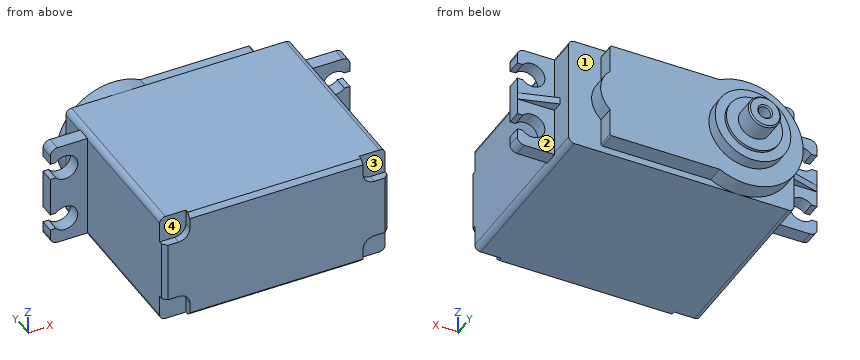
```python
from build123d import *

# Parameters (mm, degrees)
BOSS_EXTRUDE1_DEPTH = 33.6042
CUT_EXTRUDE1_DEPTH  = 1.397
CHAMFER1_SIZE       = 0.762
SKETCH3_W           = 18.6436
SKETCH3_H           = 2.4892
BOSS_EXTRUDE2_DEPTH = 6.604
SKETCH4_W           = 18.6436
SKETCH4_H           = 2.4892
BOSS_EXTRUDE3_DEPTH = 6.604
FILLET1_R           = 1.27
CUT_EXTRUDE2_DEPTH  = 3.048
SKETCH6_W           = 6.604
SKETCH6_H           = 1.2192
BOSS_EXTRUDE4_DEPTH = 1.905
CUT_EXTRUDE3_DEPTH  = 1.905
BOSS_EXTRUDE5_DEPTH = 3.0988
SKETCH9_R           = 6.731
BOSS_EXTRUDE6_DEPTH = 2.159
SKETCH10_R          = 4.9911
BOSS_EXTRUDE7_DEPTH = 0.508
SKETCH11_R          = 2.8702
BOSS_EXTRUDE8_DEPTH = 3.6576
SKETCH12_R          = 1.0668
CUT_EXTRUDE4_DEPTH  = 5.08
CHAMFER2_SIZE       = 0.254


with BuildPart() as part:
    # Sketch1 → Boss-Extrude1 (new body)
    with BuildSketch(Plane(origin=(0, 0, 0), x_dir=(1, 0, 0), z_dir=(0, 1, 0))):
        with BuildLine():
            Line((0, 9.0424), (0, -9.0424))
            ThreePointArc((0, -9.0424), (0.29757951, -9.76082049), (1.016, -10.0584))
            Line((1.016, -10.0584), (39.116, -10.0584))
            ThreePointArc((39.116, -10.0584), (39.83442049, -9.76082049), (40.132, -9.0424))
            Line((40.132, -9.0424), (40.132, 9.0424))
            ThreePointArc((40.132, 9.0424), (39.83442049, 9.76082049), (39.116, 10.0584))
            Line((39.116, 10.0584), (1.016, 10.0584))
            ThreePointArc((1.016, 10.0584), (0.29757951, 9.76082049), (0, 9.0424))
        make_face()
    extrude(amount=BOSS_EXTRUDE1_DEPTH)

    # Sketch2 → Cut-Extrude1 (cut)
    with BuildSketch(Plane.XZ):
        with BuildLine():
            Line((4.6482, 10.0584), (4.6482, 7.3533))
            ThreePointArc((4.6482, 7.3533), (4.067919955, 5.952380045), (2.667, 5.3721))
            Line((2.667, 5.3721), (0, 5.3721))
            Line((0, 5.3721), (0, 9.0424))
            ThreePointArc((0, 9.0424), (0.29757951, 9.76082049), (1.016, 10.0584))
            Line((1.016, 10.0584), (4.6482, 10.0584))
        make_face()
        with BuildLine():
            Line((35.4838, 10.0584), (35.4838, 7.3533))
            ThreePointArc((35.4838, 7.3533), (36.064080045, 5.952380045), (37.465, 5.3721))
            Line((37.465, 5.3721), (40.132, 5.3721))
            Line((40.132, 5.3721), (40.132, 9.0424))
            ThreePointArc((40.132, 9.0424), (39.83442049, 9.76082049), (39.116, 10.0584))
            Line((39.116, 10.0584), (35.4838, 10.0584))
        make_face()
        with BuildLine():
            Line((0, -5.3721), (2.667, -5.3721))
            ThreePointArc((2.667, -5.3721), (4.067919955, -5.952380045), (4.6482, -7.3533))
            Line((4.6482, -7.3533), (4.6482, -10.0584))
            Line((4.6482, -10.0584), (1.016, -10.0584))
            ThreePointArc((1.016, -10.0584), (0.29757951, -9.76082049), (0, -9.0424))
            Line((0, -9.0424), (0, -5.3721))
        make_face()
        with BuildLine():
            Line((37.465, -5.3721), (40.132, -5.3721))
            Line((40.132, -5.3721), (40.132, -9.0424))
            ThreePointArc((40.132, -9.0424), (39.83442049, -9.76082049), (39.116, -10.0584))
            Line((39.116, -10.0584), (35.4838, -10.0584))
            Line((35.4838, -10.0584), (35.4838, -7.3533))
            ThreePointArc((35.4838, -7.3533), (36.064080045, -5.952380045), (37.465, -5.3721))
        make_face()
    extrude(amount=-CUT_EXTRUDE1_DEPTH, mode=Mode.SUBTRACT)

    # Chamfer1
    chamfer1_edges = [part.edges().sort_by_distance(p)[0] for p in [
        (20.066, 0, 10.0584),
        (0, 0, 0),
        (40.132, 0, 0),
        (20.066, 0, -10.0584),
    ]]
    chamfer(chamfer1_edges, length=CHAMFER1_SIZE)

    # Sketch3 → Boss-Extrude2 (add, symmetric)
    with BuildSketch(Plane(origin=(40.132, 0, 0), x_dir=(0, 0, -1), z_dir=(1, 0, 0))):
        with Locations((0, 27.4574)):
            Rectangle(SKETCH3_W, SKETCH3_H)
    extrude(amount=BOSS_EXTRUDE2_DEPTH, both=True)

    # Sketch4 → Boss-Extrude3 (add, symmetric)
    with BuildSketch(Plane.ZY):
        with Locations((0, 27.4574)):
            Rectangle(SKETCH4_W, SKETCH4_H)
    extrude(amount=BOSS_EXTRUDE3_DEPTH, both=True)

    # Fillet1
    fillet1_edges = [part.edges().sort_by_distance(p)[0] for p in [
        (46.736, 27.4574, 9.3218),
        (46.736, 27.4574, -9.3218),
        (-6.604, 27.4574, -9.3218),
        (-6.604, 27.4574, 9.3218),
    ]]
    fillet(fillet1_edges, radius=FILLET1_R)

    # Sketch5 → Cut-Extrude2 (cut)
    with BuildSketch(Plane(origin=(0, 28.702, 0), x_dir=(1, 0, 0), z_dir=(0, 1, 0))):
        with BuildLine():
            Line((-6.604, 3.4925), (-5.625185736, 3.4925))
            ThreePointArc((-5.625185736, 3.4925), (-1.7018, 4.9911), (-5.625185736, 6.4897))
            Line((-5.625185736, 6.4897), (-6.604, 6.4897))
            Line((-6.604, 6.4897), (-6.604, 3.4925))
        make_face()
        with BuildLine():
            Line((-6.604, -6.4897), (-5.625185736, -6.4897))
            ThreePointArc((-5.625185736, -6.4897), (-1.7018, -4.9911), (-5.625185736, -3.4925))
            Line((-5.625185736, -3.4925), (-6.604, -3.4925))
            Line((-6.604, -3.4925), (-6.604, -6.4897))
        make_face()
        with BuildLine():
            Line((45.757185736, -6.4897), (46.736, -6.4897))
            Line((46.736, -6.4897), (46.736, -3.4925))
            Line((46.736, -3.4925), (45.757185736, -3.4925))
            ThreePointArc((45.757185736, -3.4925), (41.8338, -4.9911), (45.757185736, -6.4897))
        make_face()
        with BuildLine():
            Line((45.757185736, 3.4925), (46.736, 3.4925))
            Line((46.736, 3.4925), (46.736, 6.4897))
            Line((46.736, 6.4897), (45.757185736, 6.4897))
            ThreePointArc((45.757185736, 6.4897), (41.8338, 4.9911), (45.757185736, 3.4925))
        make_face()
    extrude(amount=-CUT_EXTRUDE2_DEPTH, mode=Mode.SUBTRACT)

    # Sketch6 → Boss-Extrude4 (add)
    with BuildSketch(Plane(origin=(0, 28.702, 0), x_dir=(1, 0, 0), z_dir=(0, 1, 0))):
        with Locations((-3.302, 0)):
            Rectangle(SKETCH6_W, SKETCH6_H)
        with Locations((43.434, 0)):
            Rectangle(SKETCH6_W, SKETCH6_H)
    extrude(amount=BOSS_EXTRUDE4_DEPTH)

    # Sketch7 → Cut-Extrude3 (cut)
    with BuildSketch(Plane.XY.offset(0.6096)):
        Polygon((40.132, 30.607), (46.736, 28.702), (46.736, 30.607), align=None)
        Polygon((0, 30.607), (-6.604, 28.702), (-6.604, 30.607), align=None)
    extrude(amount=-CUT_EXTRUDE3_DEPTH, mode=Mode.SUBTRACT)

    # Sketch8 → Boss-Extrude5 (add)
    with BuildSketch(Plane(origin=(0, 33.6042, 0), x_dir=(1, 0, 0), z_dir=(0, 1, 0))):
        with BuildLine():
            Line((14.8583952, -8.8392), (34.1122, -8.8392))
            ThreePointArc((34.1122, -8.8392), (34.291805122, -8.764805122), (34.3662, -8.5852))
            Line((34.3662, -8.5852), (34.3662, -3.741254719))
            ThreePointArc((34.3662, -3.741254719), (36.053651663, 0), (34.3662, 3.741254719))
            Line((34.3662, 3.741254719), (34.3662, 8.5852))
            ThreePointArc((34.3662, 8.5852), (34.291805122, 8.764805122), (34.1122, 8.8392))
            Line((34.1122, 8.8392), (14.8583952, 8.8392))
            ThreePointArc((14.8583952, 8.8392), (0, 0), (14.8583952, -8.8392))
        make_face()
    extrude(amount=BOSS_EXTRUDE5_DEPTH)

    # Sketch9 → Boss-Extrude6 (add)
    with BuildSketch(Plane(origin=(0, 36.703, 0), x_dir=(1, 0, 0), z_dir=(0, 1, 0))):
        with Locations(Location((10.0584, 0, 0), (0, 0, 270))):
            Circle(SKETCH9_R)
    extrude(amount=BOSS_EXTRUDE6_DEPTH)

    # Sketch10 → Boss-Extrude7 (add)
    with BuildSketch(Plane(origin=(0, 38.862, 0), x_dir=(1, 0, 0), z_dir=(0, 1, 0))):
        with Locations(Location((10.0584, 0, 0), (0, 0, 270))):
            Circle(SKETCH10_R)
    extrude(amount=BOSS_EXTRUDE7_DEPTH)

    # Sketch11 → Boss-Extrude8 (add)
    with BuildSketch(Plane(origin=(0, 39.37, 0), x_dir=(1, 0, 0), z_dir=(0, 1, 0))):
        with Locations(Location((10.0584, 0, 0), (0, 0, 270))):
            Circle(SKETCH11_R)
    extrude(amount=BOSS_EXTRUDE8_DEPTH)

    # Sketch12 → Cut-Extrude4 (cut)
    with BuildSketch(Plane(origin=(0, 43.0276, 0), x_dir=(1, 0, 0), z_dir=(0, 1, 0))):
        with Locations(Location((10.0584, 0, 0), (0, 0, 270))):
            Circle(SKETCH12_R)
    extrude(amount=-CUT_EXTRUDE4_DEPTH, mode=Mode.SUBTRACT)

    # Chamfer2
    chamfer2_edges = [part.edges().sort_by_distance(p)[0] for p in [
        (10.0584, 43.0276, -2.8702),
        (10.0584, 43.0276, -1.0668),
    ]]
    chamfer(chamfer2_edges, length=CHAMFER2_SIZE)


solid = part.part
```
Check sheet for the modelled part. Datum: model origin and axes. Units: mm. Face numbers are marked on the shaded views. A direction names the side the tool comes from. Round coordinates to 2 decimals unless told otherwise and drop trailing zeros. Write each loop counter-clockwise with the first axis right and the second up, starting at its lowest first coordinate (ties: lowest second). Pieces come first, ordered by that corner, then holes. Notation, with made-up numbers: M 5,54 L 26,54 A25 cw 26,72 Z; hole C -11.75,68 d3. An arc over 180 degrees is marked long. Write item = value, one per line. Start each with the question number.
1. Gauge pin test, flat ends, axial feed: pin 1 (2 mm diameter, centred on x = 27, z = 4.5, fed in from +Y); pin 2 (2.5 mm diameter, centred on x = 22.5, y = 35.5, fed in from -Z); pin 3 (9 mm diameter, centred on y = 20, z = 1.5, fed in from -X). Record the tip position at first contact, or that the pin passes through.
2. Section check A-A, the plane y = 21. Record the cut outline in (x, z), then the cut area to 3 significant figures.
3. Section check B-B, the plane x = 41. Record the cut outline in (y, z), then the cut area to 3 significant figures.
4. Scan lines: line 1 (X direction, y = 40, z = 0); line 2 (X direction, y = 26.5, z = -6.75); line 3 (Y direction, x = 7, z = 2.5). Record each from-to range of solid material in increasing order. Write a range as [from, to].
5. Tool access check on the marked faces 1, 2, 3 and 4. Record the directions out of +Z, -Z, +X, -X, +Y, -Y that give a thin tool (end or side, any length) a straight path to the whole face; none if there is none.
Results found:
q1.pin_1 = 36.7
q1.pin_2 = -8.84
q1.pin_3 = 0
q2.outline = M 0,-9.04 A1.02 ccw 1.02,-10.06 L 39.12,-10.06 A1.02 ccw 40.13,-9.04 L 40.13,9.04 A1.02 ccw 39.12,10.06 L 1.02,10.06 A1.02 ccw 0,9.04 Z
q2.area = 806 mm^2
q3.outline = M 26.21,-9.32 L 28.7,-9.32 L 28.7,-0.61 L 30.36,-0.61 L 30.36,0.61 L 28.7,0.61 L 28.7,9.32 L 26.21,9.32 Z
q3.area = 48.4 mm^2
q4.line_1 = [7.19, 8.99], [11.13, 12.93]
q4.line_2 = [-6.6, -5.35], [-2.55, 42.68], [45.48, 46.74]
q4.line_3 = [0, 39.37]
q5.face_1 = +X, +Y
q5.face_2 = -Z, +X, +Y
q5.face_3 = +Z, +X, -Y
q5.face_4 = +Z, -X, -Y
